Autodesk Inventor part; units mm, degrees
ref_plane "YZ Plane" through (0, 0, 0) normal (1, 0, 0) x (0, 1, 0)
ref_plane "XZ Plane" through (0, 0, 0) normal (0, 1, 0) x (-1, 0, 0)
ref_plane "XY Plane" through (0, 0, 0) normal (0, 0, 1) x (1, 0, 0)
sketch "Sketch1" plane through (0, 0, 0) normal (1, 0, 0) x (0, 1, 0)
  line L0 (0, 0) -> (14, 0)
  line L1 (14, 0) -> (14, -20)
  line L2 (14, -20) -> (0, -20)
  line L3 (0, -20) -> (0, 0)
  line L4 (14, -10) -> (0, -10)
  point P0 (11, -3)
  point P1 (3, -3)
  point P2 (11, -17)
  point P3 (3, -17)
  dimension "d0" = 14
  dimension "d1" = 20
  dimension "d2" = 8
  dimension "d3" = 3
  dimension "d4" = 3
  dimension "d5" = 3
extrude "Extrusion1" add sketch "Sketch1" along normal blind 2
hole "Hole1" at (0, 11, -3) at (0, 3, -3) at (0, 11, -17) at (0, 3, -17) direction (1, 0, 0) diameter 3 depth 80.45
fillet "Fillet1" radius 1.25 4 edges at (1, 14, 0) (1, 14, -20) (1, 0, -20) (1, 0, 0)
properties part number "belt_holder_2" material "アルミニウム 6061"
Geometry: final body of the model. Coordinates: model frame, mm. Give positions to 0.01 mm unless a question says otherwise; leave off trailing zeros. Write each loop counter-clockwise with the first axis right and the second up, starting at its lowest first coordinate (ties: lowest second). Pieces come first, ordered by that corner, then holes.
(1) Mould query, pull axis Y, two halves, no side actions, for faces 1 (the flat face through (1, 7, 0)), 2 (the cylindrical face through (1.01, 12.33, -2.31)), 3 (the cylindrical face through (1.014, 13.624, -19.644)). Classes: released by +Y, released by -Y, zero draft, split by the parting line, or undercut.
(2) Cut plane A-A, the plane y = 11. Return loops of the section in (x, z).
(3) Cut plane B-B, the plane z = -3. Return loops of the section in (x, y), then the cut area to 3 significant figures.
(4) Cut plane C-C, the plane x = 0.65. Return loops of the section in (y, z).
(5) First-contact query: P1, Ø5, axis at y = 11, z = -3, coming from the +X side. Flat tip, straight axial feed; report the tip coordinate or a pass-through.
(6) Ray query, line 1 (Z direction, x = 0.5, y = 3); line 2 (Y direction, x = 1.05, z = -17); line 3 (Z direction, x = 1.45, y = 3.5). Return the intervals inside material, ascending.
Values follow:
1. face 1: zero draft
1. face 2: undercut
1. face 3: released by +Y
2. outline: (0, -20) - (2, -20) - (2, -18.5) - (0, -18.5) - close; (0, -15.5) - (2, -15.5) - (2, -4.5) - (0, -4.5) - close; (0, -1.5) - (2, -1.5) - (2, 0) - (0, 0) - close
3. outline: (0, 0) - (2, 0) - (2, 1.5) - (0, 1.5) - close; (0, 4.5) - (2, 4.5) - (2, 9.5) - (0, 9.5) - close; (0, 12.5) - (2, 12.5) - (2, 14) - (0, 14) - close
3. area: 16.0 mm2
4. outline: (0, -18.75) arc R1.25 ccw to (1.25, -20) - (12.75, -20) arc R1.25 ccw to (14, -18.75) - (14, -1.25) arc R1.25 ccw to (12.75, 0) - (1.25, 0) arc R1.25 ccw to (0, -1.25) - close; hole circle Ø3 at (3, -17); hole circle Ø3 at (3, -3); hole circle Ø3 at (11, -17); hole circle Ø3 at (11, -3)
5. P1: stops at x = 2
6. line 1: z = -20 to -18.5, -15.5 to -4.5, -1.5 to 0
6. line 2: y = 0 to 1.5, 4.5 to 9.5, 12.5 to 14
6. line 3: z = -20 to -18.41, -15.59 to -4.41, -1.59 to 0
